Read the model definition and answer for the solid it produces. Units are mm, in the model's axes. Face numbers are marked on the shaded views. A direction names the side the tool comes from. Round coordinates to 2 decimals unless told otherwise and drop trailing zeros. Order: outer loops, then holes, each group sorted by start corner. A loop starts at its lowest first (then second) coordinate and runs counter-clockwise, first axis right, second up. Notation, with made-up numbers: (-15, -21.5) -> (27, -21.5) arc R31 ccw to (27, 14.5) -> close; hole circle Ø5 at (70, 79). An arc over 180 degrees is marked (long way). Answer as a JSON object with one key per item and string values. Group by question number.
Item 1: Section D-D, the plane x = -33 is taken. Write down the section's boundary in (y, z).
Item 2: Section B-B, the plane z = -11.5 is taken. Write down the section's boundary in (x, y), plus the area to 3 significant figures.
Item 3: The mould has two halves that part along Y. Classify the marked faces 1, 2 and 3: pulls with the +Y half, pulls with the -Y half, needs draft (parallel to the pull), parting line crosses it, or undercut.
Item 4: Consider probe 1 along Z at (x, y) = (0, 3); probe 2 along Z at (x, y) = (-14, 65.5); probe 3 along Y at (x, z) = (-41, -11.5). Determine where each line is inside the solid, lowest interval first. Write a range as from..to.
Item 5: Section C-C, the plane y = 26 is taken. Write down the section's boundary in (x, z), plus the area to 3 significant figures.
Item 6: Section A-A, the plane y = 73 is taken. Write down the section's boundary in (x, z).
Item 7: Given P1, Ø8, axis at x = -8.5, y = 38, coming from the -Z side; P2, Ø6, axis at y = 75, z = -11.5, coming from the -X side; P3, Ø4, axis at x = -5, y = 79.5, coming from the +Z side, each flat-ended and moving along its own axis, determine where each tip first touches the part or whether it passes through.
Item 8: For the marked faces 4, 5 and 6, determine the directions among +Z, -Z, +X, -X, +Y, -Y from which every point of the face is accessible in a straight line to the end or side of a thin tool.
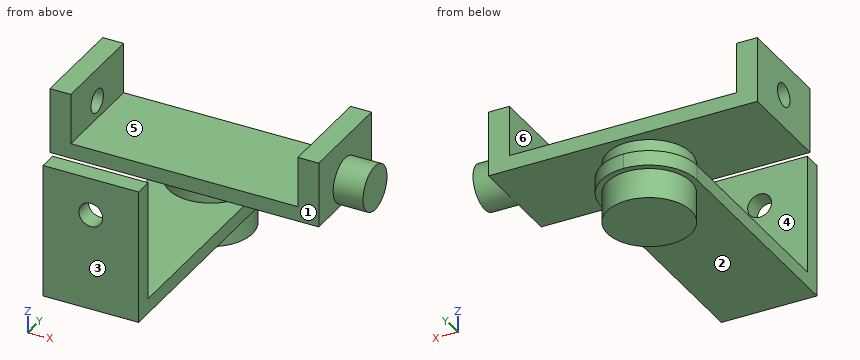
from build123d import *

# Parameters (mm, degrees)
SKETCH1_W                = 32
SKETCH1_H                = 45
SKETCH1_R                = 4
BOSS_EXTRUDE1_DEPTH      = 6
SKETCH2_W                = 32
SKETCH2_H                = 5
BOSS_EXTRUDE2_DEPTH      = 85
CUT_EXTRUDE1_DEPTH       = 85
BOSS_EXTRUDE4_DEPTH      = 5
BOSS_EXTRUDE4_DEPTH_BACK = 15
SKETCH5_W                = 90
SKETCH5_H                = 33
BOSS_EXTRUDE5_DEPTH      = 5
SKETCH6_W                = 7
SKETCH6_H                = 33
BOSS_EXTRUDE6_DEPTH      = 17
SKETCH7_R                = 7.5
BOSS_EXTRUDE7_DEPTH      = 10
SKETCH8_R                = 3.894699497
CUT_EXTRUDE2_DEPTH       = 10


with BuildPart() as part:
    # Sketch1 → Boss-Extrude1 (new body)
    with BuildSketch(Plane(origin=(0, 0, 0), x_dir=(1, 0, 0), z_dir=(0, 1, 0))):
        with Locations((0, 10)):
            Rectangle(SKETCH1_W, SKETCH1_H)
        Circle(SKETCH1_R, mode=Mode.SUBTRACT)
    extrude(amount=BOSS_EXTRUDE1_DEPTH)

    # Sketch2 → Boss-Extrude2 (add)
    with BuildSketch(Plane(origin=(0, 6, 0), x_dir=(1, 0, 0), z_dir=(0, 1, 0))):
        with Locations((0, 30)):
            Rectangle(SKETCH2_W, SKETCH2_H)
    extrude(amount=BOSS_EXTRUDE2_DEPTH)

    # Sketch3 → Cut-Extrude1 (cut)
    with BuildSketch(Plane.XY.offset(-27.5)):
        with BuildLine():
            Line((-16, 91), (-16, 75))
            ThreePointArc((-16, 75), (-11.313708499, 86.313708499), (0, 91))
            Line((0, 91), (-16, 91))
        make_face()
        with BuildLine():
            ThreePointArc((0, 91), (11.313708499, 86.313708499), (16, 75))
            Line((16, 75), (16, 91))
            Line((16, 91), (0, 91))
        make_face()
    extrude(amount=-CUT_EXTRUDE1_DEPTH, mode=Mode.SUBTRACT)

    # Sketch4 → Boss-Extrude4 (add, two sides)
    with BuildSketch(Plane.XY.offset(-27.5)) as boss_extrude4_sk:
        with BuildLine():
            ThreePointArc((14, 75), (0, 89), (-14, 75))
            Line((-14, 75), (14, 75))
        make_face()
        with BuildLine():
            Line((14, 75), (-14, 75))
            ThreePointArc((-14, 75), (0, 61), (14, 75))
        make_face()
    extrude(amount=BOSS_EXTRUDE4_DEPTH)
    extrude(boss_extrude4_sk.sketch, amount=-BOSS_EXTRUDE4_DEPTH_BACK)

    # Sketch5 → Boss-Extrude5 (add)
    with BuildSketch(Plane.XY.offset(-22.5)):
        with Locations((0, 75)):
            Rectangle(SKETCH5_W, SKETCH5_H)
    extrude(amount=BOSS_EXTRUDE5_DEPTH)

    # Sketch6 → Boss-Extrude6 (add)
    with BuildSketch(Plane.XY.offset(-17.5)):
        with Locations((-41.5, 75)):
            Rectangle(SKETCH6_W, SKETCH6_H)
        with Locations((41.5, 75)):
            Rectangle(SKETCH6_W, SKETCH6_H)
    extrude(amount=BOSS_EXTRUDE6_DEPTH)

    # Sketch7 → Boss-Extrude7 (add)
    with BuildSketch(Plane(origin=(45, 0, 0), x_dir=(0, 0, -1), z_dir=(1, 0, 0))):
        with Locations((15, 75)):
            Circle(SKETCH7_R)
    extrude(amount=BOSS_EXTRUDE7_DEPTH)

    # Sketch8 → Cut-Extrude2 (cut)
    with BuildSketch(Plane.ZY.offset(45)):
        with Locations((-11.5, 75)):
            Circle(SKETCH8_R)
    extrude(amount=-CUT_EXTRUDE2_DEPTH, mode=Mode.SUBTRACT)


solid = part.part
Values found:
{
 "1": {"outline": "(58.5, -22.5) -> (91.5, -22.5) -> (91.5, -17.5) -> (58.5, -17.5) -> close"},
 "2": {"outline": "(-45, 58.5) -> (-38, 58.5) -> (-38, 71.11) -> (-45, 71.11) -> close; (-45, 78.89) -> (-38, 78.89) -> (-38, 91.5) -> (-45, 91.5) -> close; (-16, 0) -> (16, 0) -> (16, 6) -> (-16, 6) -> close; (38, 58.5) -> (45, 58.5) -> (45, 68.37) -> (55, 68.37) -> (55, 81.63) -> (45, 81.63) -> (45, 91.5) -> (38, 91.5) -> close", "area": "732 mm2"},
 "3": {"face 1": "undercut", "face 2": "needs draft", "face 3": "pulls with the -Y half"},
 "4": {"probe 1": "-32.5..-4, 4..12.5", "probe 2": "-32.5..-27.5, -22.5..-17.5", "probe 3": "58.5..71.11, 78.89..91.5"},
 "5": {"outline": "(-16, -32.5) -> (16, -32.5) -> (16, -27.5) -> (-16, -27.5) -> close", "area": "160 mm2"},
 "6": {"outline": "(-45, -22.5) -> (-13.86, -22.5) -> (-13.86, -27.5) -> (-16, -27.5) -> (-16, -32.5) -> (-13.86, -32.5) -> (-13.86, -42.5) -> (13.86, -42.5) -> (13.86, -32.5) -> (16, -32.5) -> (16, -27.5) -> (13.86, -27.5) -> (13.86, -22.5) -> (45, -22.5) -> (45, -22.23) -> (55, -22.23) -> (55, -7.77) -> (45, -7.77) -> (45, -0.5) -> (38, -0.5) -> (38, -17.5) -> (-38, -17.5) -> (-38, -14.84) -> (-45, -14.84) -> close; (-45, -8.16) -> (-38, -8.16) -> (-38, -0.5) -> (-45, -0.5) -> close"},
 "7": {"P1": "z = -32.5", "P2": "x = 38", "P3": "z = -17.5"},
 "8": {"face 4": "+Z, +X, -X", "face 5": "+Z, +Y", "face 6": "+Z, +Y, -Y"}
}
